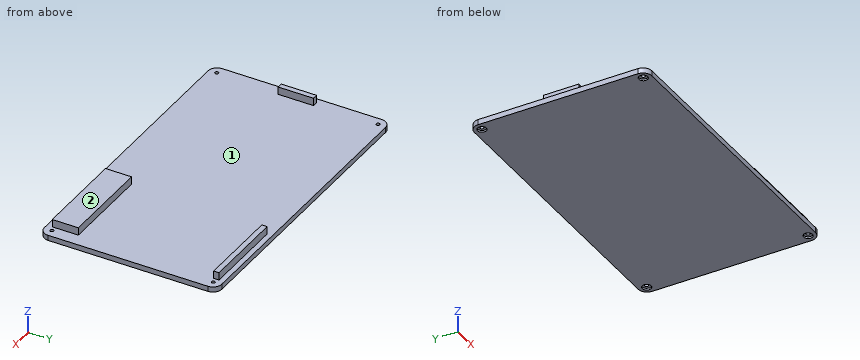
Autodesk Fusion 360 part; units mm, degrees
sketch "Sketch1" plane through (0, 0, 0) normal (0, 0, 1) x (1, 0, 0)
  line L0 (5, 0) -> (165, 0)
  line L1 (170, 5) -> (170, 95)
  line L2 (165, 100) -> (5, 100)
  line L3 (0, 95) -> (0, 5)
  arc A0 (0, 5) -> (5, 0) centre (5, 5) ccw
  arc A1 (5, 100) -> (0, 95) centre (5, 95) ccw
  arc A2 (170, 95) -> (165, 100) centre (165, 95) ccw
  arc A3 (165, 0) -> (170, 5) centre (165, 5) ccw
  point P0 (170, 0)
  point P1 (0, 100)
  dimension "d1" = 170
  dimension "d2" = 100
  dimension "d3" = 5
  dimension "d4" = 5
  dimension "d5" = 5
  dimension "d6" = 5
extrude "Extrude1" add sketch "Sketch1" along normal blind 3
sketch "Sketch2" plane through (0, 0, 3) normal (0, 0, 1) x (-1, 0, 0)
  arc A0 (-165, 0) -> (-170, -5) centre (-165, -5) ccw
  line L0 (-170, -5) -> (-170, -95)
  arc A1 (-170, -95) -> (-165, -100) centre (-165, -95) ccw
  line L1 (-165, -100) -> (-5, -100)
  arc A2 (-5, -100) -> (0, -95) centre (-5, -95) ccw
  line L2 (0, -95) -> (0, -5)
  arc A3 (0, -5) -> (-5, 0) centre (-5, -5) ccw
  line L3 (-5, 0) -> (-165, 0)
  line L4 (-3, -95) -> (-3, -5)
  arc A4 (-3, -5) -> (-5, -3) centre (-5, -5) ccw
  line L5 (-5, -3) -> (-165, -3)
  arc A5 (-165, -3) -> (-167, -5) centre (-165, -5) ccw
  line L6 (-167, -5) -> (-167, -95)
  arc A6 (-167, -95) -> (-165, -97) centre (-165, -95) ccw
  arc A7 (-5, -97) -> (-3, -95) centre (-5, -95) ccw
  line L7 (-7.5, -92.5) -> (-7.5, -7.5)
  line L8 (-7.5, -7.5) -> (-110.5, -7.5)
  line L9 (-162.5, -7.5) -> (-162.5, -92.5)
  line L10 (-162.5, -92.5) -> (-7.5, -92.5)
  line L11 (-162.5, -92.5) -> (-162.5, -97)
  line L12 (-162.5, -92.5) -> (-98.5, -92.5)
  line L13 (-98.5, -92.5) -> (-98.5, -97)
  line L14 (-115.5, -97) -> (-162.5, -97)
  line L15 (-162.5, -97) -> (-162.5, -92.5)
  line L16 (-162.5, -7.5) -> (-162.5, -3)
  line L17 (-162.5, -3) -> (-110.5, -3)
  line L18 (-110.5, -3) -> (-110.5, -14.36)
  line L19 (-110.5, -14.36) -> (-162.5, -14.36)
  line L20 (-162.5, -14.36) -> (-162.5, -3)
  line L21 (-115.5, -97) -> (-162.5, -97)
  line L22 (-162.5, -97) -> (-162.5, -94)
  line L23 (-162.5, -94) -> (-115.5, -94)
  line L24 (-98.5, -94) -> (-98.5, -97)
  line L25 (-162.5, -94) -> (-115.5, -94)
  line L26 (-115.5, -94) -> (-115.5, -97)
  line L27 (-115.5, -97) -> (-162.5, -97)
  line L28 (-162.5, -97) -> (-162.5, -94)
  line L29 (-165, -97) -> (-115.5, -97)
  line L30 (-98.5, -97) -> (-5, -97)
  dimension "d11" = 64
  dimension "d12" = 52
  dimension "d13" = 11.36
  dimension "d14" = 3
  dimension "d15" = 47
extrude "Extrude2" add sketch "Sketch2" along normal blind 4.3 contours L5 L9 L16 L17 L18 L19 L20 | L11 L14 L15 L21 L22 L23 L25 L26 L27 L28 L29
sketch "Sketch3" plane through (0, 0, 3) normal (0, 0, 1) x (-1, 0, 0)
  line L0 (-162.5, -97) -> (-162.5, -94)
  line L1 (-162.5, -94) -> (-115.5, -94)
  line L2 (-115.5, -94) -> (-115.5, -97)
  line L3 (-115.5, -97) -> (-162.5, -97)
  line L4 (-162.5, -14.36) -> (-162.5, -3)
  line L5 (-162.5, -3) -> (-110.5, -3)
  line L6 (-110.5, -3) -> (-110.5, -14.36)
  line L7 (-110.5, -14.36) -> (-162.5, -14.36)
  arc A0 (-165, 0) -> (-170, -5) centre (-165, -5) ccw
  line L8 (-170, -5) -> (-170, -95)
  arc A1 (-170, -95) -> (-165, -100) centre (-165, -95) ccw
  line L9 (-165, -100) -> (-5, -100)
  arc A2 (-5, -100) -> (0, -95) centre (-5, -95) ccw
  line L10 (0, -95) -> (0, -5)
  arc A3 (0, -5) -> (-5, 0) centre (-5, -5) ccw
  line L11 (-5, 0) -> (-165, 0)
sketch "Sketch4" plane through (0, 0, 3) normal (0, 0, 1) x (1, 0, 0)
extrude "Extrude3" add 1 faces at (127.8333, 14.36, 4.4333) along direction (0, 1, 0) blind 3.34
sketch "Sketch5" plane through (0, 0, 3) normal (0, 0, 1) x (-1, 0, 0)
sketch "Sketch6" plane through (0, 0, 3) normal (0, 0, 1) x (-1, 0, 0)
  circle A0 centre (-4.5302, -4.5302) radius 1
  circle A1 centre (-4.5302, -95.4698) radius 1
  circle A2 centre (-165.4698, -95.4698) radius 1
  circle A3 centre (-165.4698, -4.5302) radius 1
  dimension "d26" = 2
  dimension "d30" = 2
  dimension "d34" = 2
  dimension "d38" = 2
extrude "Extrude4" cut sketch "Sketch6" against normal blind 3
sketch "Sketch7" plane through (0, 0, 0) normal (0, 0, -1) x (1, 0, 0)
  circle A0 centre (4.5302, -95.4698) radius 1
  circle A1 centre (165.4698, -95.4698) radius 1
  circle A2 centre (4.5302, -4.5302) radius 1
  circle A3 centre (165.4698, -4.5302) radius 1
  arc A4 (170, -5) -> (165, 0) centre (165, -5) ccw
  line L0 (165, 0) -> (5, 0)
  arc A5 (5, 0) -> (0, -5) centre (5, -5) ccw
  line L1 (0, -5) -> (0, -95)
  arc A6 (0, -95) -> (5, -100) centre (5, -95) ccw
  line L2 (5, -100) -> (165, -100)
  arc A7 (165, -100) -> (170, -95) centre (165, -95) ccw
  line L3 (170, -95) -> (170, -5)
  circle A8 centre (4.5302, -4.5302) radius 2.5
  circle A9 centre (4.5302, -95.4698) radius 2.5
  circle A10 centre (165.4698, -95.4698) radius 2.5
  circle A11 centre (165.4698, -4.5302) radius 2.5
  dimension "d41" = 1.5
  dimension "d42" = 1.5
  dimension "d43" = 1.5
  dimension "d44" = 1.5
extrude "Extrude5" cut sketch "Sketch7" against normal blind 1 contours A8 | A9 | A10 | A11
sketch "Sketch8" plane through (0, 0, 3) normal (0, 0, 1) x (1, 0, 0)
sketch "Sketch9" plane through (0, 0, 3) normal (0, 0, 1) x (-1, 0, 0)
  line L0 (-3, -40) -> (-6, -40)
  line L1 (-6, -40) -> (-6, -60)
  line L2 (-6, -60) -> (-3, -60)
  line L3 (-3, -60) -> (-3, -40)
  point P0 (-4.5, -50)
  dimension "d51" = 3
  dimension "d52" = 20
extrude "Extrude6" add sketch "Sketch9" along normal blind 4.3
The listing builds one solid part. Answer for the finished solid, in the listing's coordinates (mm). Face numbers are marked on the shaded views. Give positions to 0.01 mm unless a question says otherwise; leave off trailing zeros. Write each loop counter-clockwise with the first axis right and the second up, starting at its lowest first coordinate (ties: lowest second). Pieces come first, ordered by that corner, then holes. Notation, with made-up numbers: (-6, 63.5) - (21, 63.5) arc R17 ccw to (21, 86.5) - close; hole circle Ø7 at (-13, 72). An arc over 180 degrees is marked (long way). Use one line per item in the form item = value. Start each with the question number.
1) Find section D-D on y = 31. Determine the outline of the cut face in (x, z).
2) The mould has two halves that part along Y. Classify the marked faces 1 and 2: pulls with the +Y half, pulls with the -Y half, needs draft (parallel to the pull), parting line crosses it, or undercut.
3) Find section C-C on y = 48. Determine the outline of the cut face in (x, z), plus the area to 3 significant figures.
4) Consider line 1 along Y through (x, z) = (131, 6.75); line 2 along X through (y, z) = (46, 3.25); line 3 along Z through (x, y) = (141.5, 60.5). Determine where each line is inside the solid, lowest interval first. Write a range as from..to.
5) Flat-ended cylindrical pins translate along their axes: pin 1 Ø3 at (x, y) = (4.53, 95.47) entering from +Z; pin 2 Ø3 at (x, y) = (58, 22) entering from -Z; pin 3 Ø2.5 at (x, y) = (5, 94.5) entering from -Z; pin 4 Ø3.5 at (x, z) = (4, 5.5) entering from -Y. Find the tip coordinate at first contact, or state that the pin passes through.
6) Find section B-B on x = 120. Determine the outline of the cut face in (y, z).
7) Find section A-A on z = 5.5. Determine the outline of the cut face in (x, y), plus the area to 3 significant figures.
Geometry results:
q1.outline = (0, 0) - (170, 0) - (170, 3) - (0, 3) - close
q2.face_1 = undercut
q2.face_2 = needs draft
q3.outline = (0, 0) - (170, 0) - (170, 3) - (6, 3) - (6, 7.3) - (3, 7.3) - (3, 3) - (0, 3) - close
q3.area = 523 mm2
q4.line_1 = 3..17.7, 94..97
q4.line_2 = 3..6
q4.line_3 = 0..3
q5.pin_1 = 3
q5.pin_2 = 0
q5.pin_3 = 1
q5.pin_4 = 40
q6.outline = (0, 0) - (100, 0) - (100, 3) - (97, 3) - (97, 7.3) - (94, 7.3) - (94, 3) - (17.7, 3) - (17.7, 7.3) - (3, 7.3) - (3, 3) - (0, 3) - close
q7.outline = (3, 40) - (6, 40) - (6, 60) - (3, 60) - close; (110.5, 3) - (162.5, 3) - (162.5, 17.7) - (110.5, 17.7) - close; (115.5, 94) - (162.5, 94) - (162.5, 97) - (115.5, 97) - close
q7.area = 965 mm2
